The model under review builds one solid part; all positions refer to its coordinate system, in mm. A direction names the side the tool comes from. Coordinates: 2 decimals unless noted, no trailing zeros. Order: outer loops, then holes, each group sorted by start corner. A loop starts at its lowest first (then second) coordinate and runs counter-clockwise, first axis right, second up. Notation, with made-up numbers: (24.25, -36.5) -> (29.25, -36.5) arc R21 ccw to (29.25, 0.5) -> close; hole circle Ø4 at (-14, 8). An arc over 180 degrees is marked (long way). Use one line per item in the form item = value.
from build123d import *

# Parameters (mm, degrees)
SKETCH9_W           = 75
SKETCH9_H           = 40
BOSS_EXTRUDE5_DEPTH = 5
SKETCH10_R          = 10
SKETCH10_R_2        = 8
SKETCH10_R_3        = 2
CUT_EXTRUDE5_DEPTH  = 43.793106922
SKETCH11_R          = 1.7
CUT_EXTRUDE6_DEPTH  = 43.793106922
FILLET1_R           = 10


with BuildPart() as part:
    # Sketch9 → Boss-Extrude5 (new body)
    with BuildSketch(Plane(origin=(0, 0, 0), x_dir=(1, 0, 0), z_dir=(0, 1, 0))):
        Rectangle(SKETCH9_W, SKETCH9_H)
    extrude(amount=BOSS_EXTRUDE5_DEPTH)

    # Sketch10 → Cut-Extrude5 (cut, through all)
    # profile 1 of 12: a face of its own
    with BuildSketch(Plane(origin=(0, 5, 0), x_dir=(1, 0, 0), z_dir=(0, 1, 0))):
        with Locations((9.729894245, 0.839124812)):
            Circle(SKETCH10_R)
    # profile 2 of 12: a face of its own
    with BuildSketch(Plane(origin=(0, 5, 0), x_dir=(1, 0, 0), z_dir=(0, 1, 0))):
        Polygon((10.022213237, -9.821914184), (10.022213237, 12.178085816), (-20.977786763, 12.184810323), (-20.9811162, -9.817222635), align=None)
        with Locations((-3.270105755, 0.839124812)):
            Circle(SKETCH10_R_2, mode=Mode.SUBTRACT)
    # profile 3 of 12: a face of its own
    with BuildSketch(Plane(origin=(0, 5, 0), x_dir=(1, 0, 0), z_dir=(0, 1, 0))):
        with BuildLine():
            ThreePointArc((19.729894245, 0.839124812), (16.903567987, 7.806075726), (10.022213237, 10.834851379))
            Line((10.022213237, 10.834851379), (10.022213237, -9.156601756))
            ThreePointArc((10.022213237, -9.156601756), (16.903567987, -6.127826103), (19.729894245, 0.839124812))
        make_face()
    # profile 4 of 12: a face of its own
    with BuildSketch(Plane(origin=(0, 5, 0), x_dir=(1, 0, 0), z_dir=(0, 1, 0))):
        with BuildLine():
            Line((10.022213237, -9.156601756), (10.022213237, 10.834851379))
            ThreePointArc((10.022213237, 10.834851379), (5.474717618, 9.888626006), (1.845278861, 6.989965424))
            ThreePointArc((1.845278861, 6.989965424), (3.972928034, 4.235955914), (4.729894245, 0.839124812))
            ThreePointArc((4.729894245, 0.839124812), (3.972928034, -2.557706291), (1.845278861, -5.311715801))
            ThreePointArc((1.845278861, -5.311715801), (5.474717618, -8.210376383), (10.022213237, -9.156601756))
        make_face()
    # profile 5 of 12: a face of its own
    with BuildSketch(Plane(origin=(0, 5, 0), x_dir=(1, 0, 0), z_dir=(0, 1, 0))):
        with Locations((9.729894245, 0.839124812)):
            Circle(SKETCH10_R)
    # profile 6 of 12: a face of its own
    with BuildSketch(Plane(origin=(0, 5, 0), x_dir=(1, 0, 0), z_dir=(0, 1, 0))):
        with Locations((-3.270105755, 0.839124812)):
            Circle(SKETCH10_R_2)
    # profile 7 of 12: a face of its own
    with BuildSketch(Plane(origin=(0, 5, 0), x_dir=(1, 0, 0), z_dir=(0, 1, 0))):
        with Locations((9.729894245, 0.839124812)):
            Circle(SKETCH10_R)
    # profile 8 of 12: a face of its own
    with BuildSketch(Plane(origin=(0, 5, 0), x_dir=(1, 0, 0), z_dir=(0, 1, 0))):
        with Locations((-3.270105755, 0.839124812)):
            Circle(SKETCH10_R_2)
    # profile 9 of 12: a face of its own
    with BuildSketch(Plane(origin=(0, 5, 0), x_dir=(1, 0, 0), z_dir=(0, 1, 0))):
        with Locations(Location((24.229894245, 5.839124812, 0), (0, 0, 270))):
            Circle(SKETCH10_R_3)
    # profile 10 of 12: a face of its own
    with BuildSketch(Plane(origin=(0, 5, 0), x_dir=(1, 0, 0), z_dir=(0, 1, 0))):
        with Locations(Location((24.229894245, -4.160875188, 0), (0, 0, 270))):
            Circle(SKETCH10_R_3)
    # profile 11 of 12: a face of its own
    with BuildSketch(Plane(origin=(0, 5, 0), x_dir=(1, 0, 0), z_dir=(0, 1, 0))):
        with Locations(Location((-24.770105755, 5.839124812, 0), (0, 0, 270))):
            Circle(SKETCH10_R_3)
    # profile 12 of 12: a face of its own
    with BuildSketch(Plane(origin=(0, 5, 0), x_dir=(1, 0, 0), z_dir=(0, 1, 0))):
        with Locations(Location((-24.770105755, -4.160875188, 0), (0, 0, 270))):
            Circle(SKETCH10_R_3)
    extrude(amount=-CUT_EXTRUDE5_DEPTH, mode=Mode.SUBTRACT)

    # Sketch11 → Cut-Extrude6 (cut, through all)
    with BuildSketch(Plane(origin=(0, 5, 0), x_dir=(1, 0, 0), z_dir=(0, 1, 0))):
        with Locations(Location((-32, 15, 0), (0, 0, 270))):
            Circle(SKETCH11_R)
        with Locations(Location((32, 15, 0), (0, 0, 270))):
            Circle(SKETCH11_R)
        with Locations(Location((32, -15, 0), (0, 0, 270))):
            Circle(SKETCH11_R)
        with Locations(Location((-32, -15, 0), (0, 0, 270))):
            Circle(SKETCH11_R)
    extrude(amount=-CUT_EXTRUDE6_DEPTH, mode=Mode.SUBTRACT)

    # Fillet1
    fillet1_edges = [part.edges().sort_by_distance(p)[0] for p in [
        (37.5, 2.5, 20),
        (-37.5, 2.5, 20),
        (-37.5, 2.5, -20),
        (37.5, 2.5, -20),
    ]]
    fillet(fillet1_edges, radius=FILLET1_R)


solid = part.part
Item 1: We need section A-A (z = -14). Write out the cut boundary in (x, y), plus the area to 3 significant figures.
Results found:
outline = (-36.67, 0) -> (-33.37, 0) -> (-33.37, 5) -> (-36.67, 5) -> close; (-30.63, 0) -> (30.63, 0) -> (30.63, 5) -> (-30.63, 5) -> close; (33.37, 0) -> (36.67, 0) -> (36.67, 5) -> (33.37, 5) -> close
area = 339 mm²
Item 2: To check wall thickness, follow L1, parallel to X at y = 3.5, z = -7; L2, parallel to Z at x = -23.5, y = 1.8; L3, parallel to Z at x = 1, y = 2.55. State the ranges of each line that lie inside material, in increasing order. Write a range as from..to.
Results found:
L1 = -37.5..-26.4, -23.14..-20.98, 17.61..22.6, 25.86..37.5
L2 = -20..-7.38, -4.29..2.62, 5.71..20
L3 = -20..-12.18, 9.82..20
Item 3: We need section D-D (z = -9). Write out the cut boundary in (x, y), plus the area to 3 significant figures.
Results found:
outline = (-37.5, 0) -> (-20.98, 0) -> (-20.98, 5) -> (-37.5, 5) -> close; (15.51, 0) -> (37.5, 0) -> (37.5, 5) -> (15.51, 5) -> close
area = 193 mm²
Item 4: Draft analysis for pull direction X (two halves, no side actions). For faces 3 (the face through (-33.5, 2.5, -14.2)), 4 (the face through (-1, 5, 13)), 5 (the face through (37.5, 2, 0)), 6 (the face through (-34.65, 2.54, 16.99)), state which applies: released by +X, released by -X, zero draft, split by the parting line, or undercut.
Results found:
face_3 = undercut
face_4 = zero draft
face_5 = released by +X
face_6 = released by -X
Item 5: We need section B-B (x = -32). Write out the cut boundary in (y, z).
Results found:
outline = (0, -18.93) -> (5, -18.93) -> (5, -16.7) -> (0, -16.7) -> close; (0, -13.3) -> (5, -13.3) -> (5, 13.3) -> (0, 13.3) -> close; (0, 16.7) -> (5, 16.7) -> (5, 18.93) -> (0, 18.93) -> close
Item 6: Tool access review of faces 1 (the face through (10.022, 3, -11)), 2 (the face through (0, 2, 20)): name each direction out of +Z, -Z, +X, -X, +Y, -Y from which nothing blocks a thin tool from reaching the whole face with its end or side.
Results found:
face_1 = +Y, -Y
face_2 = +Z, +X, -X, +Y, -Y
Item 7: We need section C-C (y = 3.05). State how many separate pieces and enclosed holes the cut face has, plus the area to 3 significant figures.
Results found:
separate_pieces = 1
enclosed_holes = 9
area = 1,990 mm²
Item 8: Clearance check with a flat-ended pin moving along its axis: pin 1 (1.5 mm diameter, centred on y = 2.5, z = -11.5, fed in from -X). State where the tip first meets the part, or that it passes through.
Results found:
pin_1 = -37.47
